from build123d import *

# Parameters (mm, degrees)
ESQUISSE1_W      = 25
ESQUISSE1_H      = 25
ESQUISSE1_R      = 1.5
ESQUISSE1_R_2    = 3
EXTRUSION3_DEPTH = 30
ESQUISSE8_R      = 10
EXTRUSION4_DEPTH = 28


with BuildPart() as part:
    # Esquisse1 → Extrusion3 (new body)
    with BuildSketch(Plane.XY):
        Rectangle(ESQUISSE1_W, ESQUISSE1_H)
        with Locations((10, 10)):
            Circle(ESQUISSE1_R, mode=Mode.SUBTRACT)
        Circle(ESQUISSE1_R_2, mode=Mode.SUBTRACT)
        with Locations((-10, 10)):
            Circle(ESQUISSE1_R, mode=Mode.SUBTRACT)
        with Locations((10, -10)):
            Circle(ESQUISSE1_R, mode=Mode.SUBTRACT)
        with Locations((-10, -10)):
            Circle(ESQUISSE1_R, mode=Mode.SUBTRACT)
    extrude(amount=EXTRUSION3_DEPTH)

    # Esquisse8 → Extrusion4 (cut)
    with BuildSketch(Plane.XY.offset(30)):
        Circle(ESQUISSE8_R)
    extrude(amount=-EXTRUSION4_DEPTH, mode=Mode.SUBTRACT)


solid = part.part
Model file for the job. Use its own axes, mm. Round coordinates to 2 decimals unless told otherwise and drop trailing zeros. Loops run counter-clockwise (first coordinate to the right, second up) from the corner with the lowest first, then second, coordinate; pieces in that order, holes last. Notation, with made-up numbers: M 38,46.5 L 79,46.5 A18 cw 79,71.5 Z; hole C 1.25,-40 d1. An arc over 180 degrees is marked long. One line per question, with ' | ' between items.
1) Band-saw the part on B-B (z = 16.5). Give the cut face in (x, y), then the cut area to 3 significant figures.
Solved:
outline: M -12.5,-12.5 L 12.5,-12.5 L 12.5,12.5 L -12.5,12.5 Z; hole C -10,-10 d3; hole C -10,10 d3; hole C 0,0 d20; hole C 10,-10 d3; hole C 10,10 d3 | area: 283 mm²
2) Band-saw the part on D-D (x = 10.5). Give the cut face in (y, z), then the cut area to 3 significant figures.
Solved:
outline: M -12.5,0 L -11.41,0 L -11.41,30 L -12.5,30 Z; M -8.59,0 L 8.59,0 L 8.59,30 L -8.59,30 Z; M 11.41,0 L 12.5,0 L 12.5,30 L 11.41,30 Z | area: 580 mm²
3) Drill centre lines: line 1 along Y through (x, z) = (0, 23.25); line 2 along X through (y, z) = (-10.5, 13). Where is each one in solid material? Low to high.
Solved:
line 1: y = -12.5 to -10, 10 to 12.5 | line 2: x = -12.5 to -11.41, -8.59 to 8.59, 11.41 to 12.5
4) Band-saw the part on A-A (x = 0). Give the cut face in (y, z).
Solved:
outline: M -12.5,0 L -3,0 L -3,2 L -10,2 L -10,30 L -12.5,30 Z; M 3,0 L 12.5,0 L 12.5,30 L 10,30 L 10,2 L 3,2 Z
5) Mould opens along X. For faces 1 (the cylindrical face through (-2.17, -9.76, 16.2)), 2 (the flat face through (-12.5, 0, 15)), 3 (the flat face through (2.1, 2.4, 2)), 4 (the flat face through (-3, 3, 0)) say: +X half, -X half, draft (parallel to the pull), parting line (faces both ways), or undercut.
Solved:
face 1: undercut | face 2: -X half | face 3: undercut | face 4: draft
6) Flat gauge pins, fed straight in: pin 1 (9.5 mm diameter, centred on x = 0, y = 0, fed in from +Z); pin 2 (2.5 mm diameter, centred on x = 10, y = -10, fed in from -Z). Where does each tip first touch, or does it go through?
Solved:
pin 1: stops at z = 2 | pin 2: passes through
7) Band-saw the part on C-C (y = 2). Give the cut face in (x, z), then the cut area to 3 significant figures.
Solved:
outline: M -12.5,0 L -2.24,0 L -2.24,2 L -9.8,2 L -9.8,30 L -12.5,30 Z; M 2.24,0 L 12.5,0 L 12.5,30 L 9.8,30 L 9.8,2 L 2.24,2 Z | area: 192 mm²
